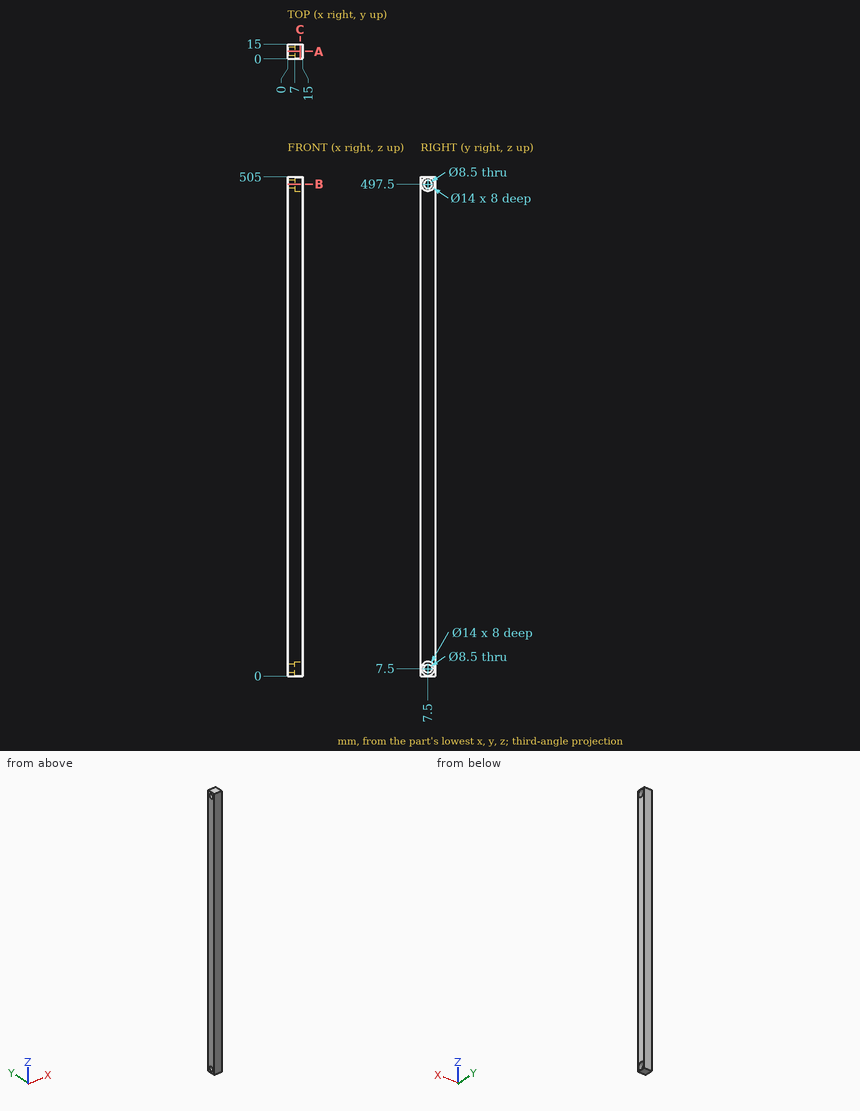
Can you work these out from the drawing? Everything is in mm from the part's minimum corner. Round coordinates to 2 decimals unless told otherwise and drop trailing zeros. Order: outer loops, then holes, each group sorted by start corner. A loop starts at its lowest first (then second) coordinate and runs counter-clockwise, first axis right, second up.
(1) If I drill on L1, parallel to Y at x = 12.25, z = 7.5; L2, parallel to Y at x = 4.5, z = 7.5; L3, parallel to Z at x = 7.25, y = 13.25, over which ranges is the centre line in solid material (lowest first)?
Results are:
L1: y = 0 to 0.5, 14.5 to 15
L2: y = 0 to 3.25, 11.75 to 15
L3: z = 0 to 3.51, 11.49 to 493.51, 501.49 to 505
(2) If we section it at A-A (y = 7.5): Please give me the cut outline in (x, z), plus the area to 3 significant figures.
Results are:
outline: (0, 0) - (15, 0) - (15, 0.5) - (7, 0.5) - (7, 3.25) - (0, 3.25) - close; (0, 11.75) - (7, 11.75) - (7, 14.5) - (15, 14.5) - (15, 490.5) - (7, 490.5) - (7, 493.25) - (0, 493.25) - close; (0, 501.75) - (7, 501.75) - (7, 504.5) - (15, 504.5) - (15, 505) - (0, 505) - close
area: 7,230 mm2
(3) I'm going to push a flat-ended pin straight in: pin 1 (1 mm diameter, centred on x = 13, z = 238.5, fed in from -Y). Where does the tip first touch, or does it pass through?
Results are:
pin 1: stops at y = 0
(4) If we section it at C-C (x = 12.5): Please give me the cut outline in (y, z).
Results are:
outline: (0, 0) - (15, 0) - (15, 505) - (0, 505) - close; hole circle Ø14 at (7.5, 7.5); hole circle Ø14 at (7.5, 497.5)
(5) If we section it at B-B (z = 497.5): Please give me the cut outline in (x, y), plus the area to 3 significant figures.
Results are:
outline: (0, 0) - (15, 0) - (15, 0.5) - (7, 0.5) - (7, 3.25) - (0, 3.25) - close; (0, 11.75) - (7, 11.75) - (7, 14.5) - (15, 14.5) - (15, 15) - (0, 15) - close
area: 53.5 mm2
